Design review of the part built by this model. Coordinates are the model's own, in mm. A direction names the side the tool comes from. Give positions to 0.01 mm unless a question says otherwise; leave off trailing zeros. Loops run counter-clockwise (first coordinate to the right, second up) from the corner with the lowest first, then second, coordinate; pieces in that order, holes last. Notation, with made-up numbers: M -39,-13 L 17,-13 A26 cw 17,19 Z; hole C 81,52 d2. An arc over 180 degrees is marked long. Use a Markdown table: item, result. Add a question column.
(1) Draft analysis for pull direction Z (two halves, no side actions). For faces 4 (the face through (-22.25, 0.04, -30.84)), 5 (the face through (32, 0, 34.925)), 6 (the face through (-25.4, 0, 21)), state which applies: pulls with the +Z half, pulls with the -Z half, needs draft (parallel to the pull), parting line crosses it, or undercut.
(2) For probe 1 along X at (y, z) = (-1, 13.5); probe 2 along X at (y, z) = (1.75, -20); probe 3 along Z at (x, y) = (-23, 1) (3 decimals), list the stretches that pass through material, from the lowest coordinate up.
(3) Add section B-B, the plane x = 24.5. Give the boundary of the cut face in (y, z) (3 decimals).
(4) For faces 1 (the face through (-32, 0, 34.925)), 2 (the face through (25.4, 0, 21)), 3 (the face through (12.7, 0, -22)), list the 3-axis set-ups (+Z, -Z, +X, -X, +Y, -Y) from which the entire face can be reached by the end or side of a thin tool; tool diameter is ignored.
(5) Add section C-C, the plane y = 0.75. Give the boundary of the cut face in (x, z) (3 decimals).
(6) Insertion check: pin 1 Ø6 at (x, z) = (-25.4, -29.845) entering from -Y; pin 2 Ø3 at (x, y) = (-1.5, -0.5) entering from -Z (3 decimals); pin 3 Ø3 at (x, y) = (-7.5, 1) entering from +Z (3 decimals). Each pin has a flat end and moves straight along its axis. Give the tip position at first contact, or say it passes through.
(7) Add section A-A, the plane z = 12.5. Give the boundary of the cut face in (x, y) (3 decimals).
```python
from build123d import *

# Parameters (mm, degrees)
SKETCH1_W           = 76.2
SKETCH1_H           = 69.85
BOSS_EXTRUDE1_DEPTH = 3.175
SKETCH2_W           = 50.8
SKETCH2_H           = 27.94
CUT_EXTRUDE1_DEPTH  = 7.35
SKETCH4_R           = 3.302
CUT_EXTRUDE2_DEPTH  = 7.35
SKETCH5_W           = 25.4
SKETCH5_H           = 25.4
CUT_EXTRUDE3_DEPTH  = 7.35


with BuildPart() as part:
    # Sketch1 → Boss-Extrude1 (new body, symmetric)
    with BuildSketch(Plane(origin=(0, 0, 0), x_dir=(1, 0, 0), z_dir=(0, 1, 0))):
        Rectangle(SKETCH1_W, SKETCH1_H)
    extrude(amount=BOSS_EXTRUDE1_DEPTH, both=True)

    # Sketch2 → Cut-Extrude1 (cut, through all)
    with BuildSketch(Plane(origin=(0, 3.175, 0), x_dir=(1, 0, 0), z_dir=(0, 1, 0))):
        with Locations((0, -20.955)):
            Rectangle(SKETCH2_W, SKETCH2_H)
    extrude(amount=-CUT_EXTRUDE1_DEPTH, mode=Mode.SUBTRACT)

    # Sketch4 → Cut-Extrude2 (cut, through all)
    with BuildSketch(Plane(origin=(0, 3.175, 0), x_dir=(1, 0, 0), z_dir=(0, 1, 0))):
        with Locations((-25.4, 29.845)):
            Circle(SKETCH4_R)
        with Locations((25.4, 29.845)):
            Circle(SKETCH4_R)
    extrude(amount=-CUT_EXTRUDE2_DEPTH, mode=Mode.SUBTRACT)

    # Sketch5 → Cut-Extrude3 (cut, through all)
    with BuildSketch(Plane(origin=(0, 3.175, 0), x_dir=(1, 0, 0), z_dir=(0, 1, 0))):
        with Locations((0, 22.225)):
            Rectangle(SKETCH5_W, SKETCH5_H)
    extrude(amount=-CUT_EXTRUDE3_DEPTH, mode=Mode.SUBTRACT)


solid = part.part
```
Established:
| question | item | result |
|---|---|---|
| 1 | face 4 | undercut |
| 1 | face 5 | pulls with the +Z half |
| 1 | face 6 | needs draft |
| 2 | probe 1 | -38.1 to -25.4, 25.4 to 38.1 |
| 2 | probe 2 | -38.1 to -12.7, 12.7 to 38.1 |
| 2 | probe 3 | -34.925 to -32.113, -27.577 to 6.985 |
| 3 | outline | M -3.175,-34.925 L 3.175,-34.925 L 3.175,-33.022 L -3.175,-33.022 Z; M -3.175,-26.668 L 3.175,-26.668 L 3.175,6.985 L -3.175,6.985 Z |
| 4 | face 1 | +Z, +X, -X, +Y, -Y |
| 4 | face 2 | +Z, +Y, -Y |
| 4 | face 3 | -Z, +Y, -Y |
| 5 | outline | M -38.1,-34.925 L -12.7,-34.925 L -12.7,-9.525 L 12.7,-9.525 L 12.7,-34.925 L 38.1,-34.925 L 38.1,34.925 L 25.4,34.925 L 25.4,6.985 L -25.4,6.985 L -25.4,34.925 L -38.1,34.925 Z; hole C -25.4,-29.845 d6.604; hole C 25.4,-29.845 d6.604 |
| 6 | pin 1 | through |
| 6 | pin 2 | z = -9.525 |
| 6 | pin 3 | z = 6.985 |
| 7 | outline | M -38.1,-3.175 L -25.4,-3.175 L -25.4,3.175 L -38.1,3.175 Z; M 25.4,-3.175 L 38.1,-3.175 L 38.1,3.175 L 25.4,3.175 Z |
